Here's the drawing with two shaded views (mm, measured from the low corner). I have some questions. Coordinates: 2 decimals unless noted, no trailing zeros. Write each loop counter-clockwise with the first axis right and the second up, starting at its lowest first coordinate (ties: lowest second). Pieces come first, ordered by that corner, then holes.
Item 1: Thinking about a two-plate mould opening in X: for the marked faces 1, 2 and 3, which applies, +X half, -X half, draft (parallel to the pull), parting line (faces both ways), or undercut?
Item 2: For P1, Ø12, axis at x = 21.1, z = 50.03, coming from the +Y side; P2, Ø2, axis at x = 76.5, y = 8.5, coming from the +Z side; P3, Ø4, axis at x = 65.5, y = 21.5, coming from the +Z side; P4, Ø5, axis at x = 118, y = 20.5, coming from the -Z side, each with a flat end and sliding along its axis, tell me the tip position at first contact or that it passes through.
Item 3: I want a section at B-B on x = 32.5. Please give me the cut outline in (y, z), then the cut area to 3 significant figures.
Item 4: I want a section at A-A on z = 19. Please give me the cut outline in (x, y) (1 decimal).
Item 5: I want a section at C-C on z = 80. Please give me the cut outline in (x, y), then the cut area to 3 significant figures.
Item 6: If I drill on probe 1 along X at (y, z) = (21.75, 29.5) (1 decimal); probe 2 along X at (y, z) = (17.75, 52.5) (1 decimal); probe 3 along X at (y, z) = (9.25, 72) (1 decimal), over which ranges is the centre line in solid material (lowest first)?
Item 7: I want a section at D-D on y = 19.25. State how many separate pieces and enclosed holes the cut face has, then the cut area to 3 significant figures.
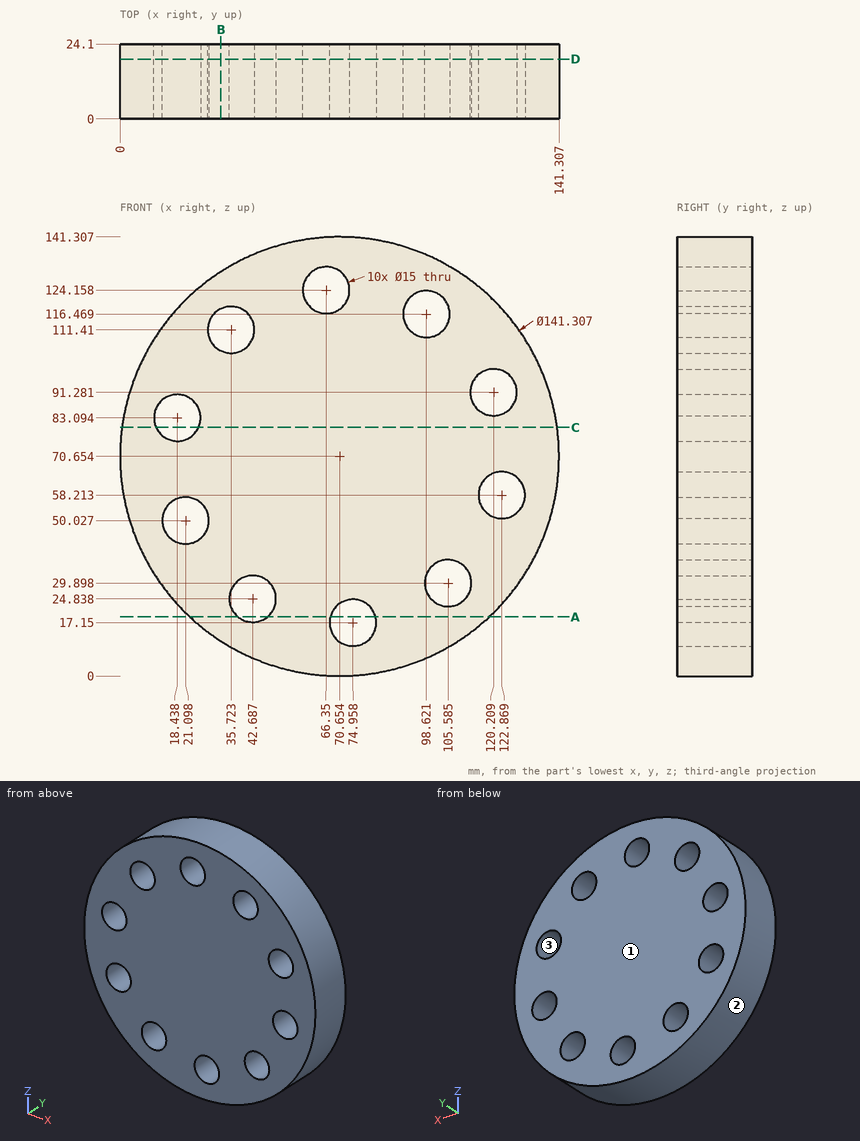
Response values:
1. face 1: draft
1. face 2: parting line
1. face 3: undercut
2. P1: passes through
2. P2: stops at z = 141.14
2. P3: stops at z = 141.24
2. P4: stops at z = 16.06
3. outline: (0, 11.19) - (24.1, 11.19) - (24.1, 104.64) - (0, 104.64) - close; (0, 118.18) - (24.1, 118.18) - (24.1, 130.12) - (0, 130.12) - close
3. area: 2,540 mm2
4. outline: (22.4, 0) - (38, 0) - (38, 24.1) - (22.4, 24.1) - close; (47.4, 0) - (67.7, 0) - (67.7, 24.1) - (47.4, 24.1) - close; (82.2, 0) - (118.9, 0) - (118.9, 24.1) - (82.2, 24.1) - close
5. outline: (0.62, 0) - (11.61, 0) - (11.61, 24.1) - (0.62, 24.1) - close; (25.27, 0) - (140.69, 0) - (140.69, 24.1) - (25.27, 24.1) - close
5. area: 3,050 mm2
6. probe 1: x = 13.2 to 36.8, 48.6 to 98.1, 113.1 to 128.1
6. probe 2: x = 2.4 to 14, 28.2 to 118, 127.7 to 138.9
6. probe 3: x = 0 to 141.3
7. separate pieces: 1
7. enclosed holes: 10
7. area: 13,900 mm2
